Verification items for the finished model (mm, model axes). A direction names the side the tool comes from. Round coordinates to 2 decimals unless told otherwise and drop trailing zeros. Order: outer loops, then holes, each group sorted by start corner. A loop starts at its lowest first (then second) coordinate and runs counter-clockwise, first axis right, second up. Notation, with made-up numbers: (21, 66) -> (32, 66) arc R19 ccw to (32, 95) -> close; hole circle Ø7 at (-9.75, 74). An arc over 180 degrees is marked (long way). Put each result on its own line as item: value.
Autodesk Inventor part; units mm, degrees
ref_plane "Work Plane1" through (-20, 20, -22) normal (0, -0.791285, -0.6114475) x (1, 0, 0)
ref_plane "YZ Plane" through (0, 0, 0) normal (1, 0, 0) x (0, 1, 0)
ref_plane "XZ Plane" through (0, 0, 0) normal (0, 1, 0) x (-1, 0, 0)
sketch "Sketch1" plane through (0, 0, 0) normal (0, 1, 0) x (-1, 0, 0)
  line L0 (0, 0) -> (20, 0)
  line L1 (20, 0) -> (20, -25)
  line L2 (20, -25) -> (0, -25)
  line L3 (0, -25) -> (0, 0)
  circle A0 centre (10, -11) radius 2.6
  line L4 (20, -25) -> (0, -25)
  line L5 (0, -25) -> (0, -22)
  line L6 (0, -22) -> (20, -22)
  line L7 (20, -22) -> (20, -25)
  line L8 (0, -22) -> (20, 0) construction
  point P0 (10, -11)
  dimension "d2" = 20
  dimension "d3" = 25
  dimension "d4" = 5.2
  dimension "d7" = 3
extrude "Extrusion1" add sketch "Sketch1" along normal blind 3
extrude "Extrusion2" add sketch "Sketch1" along normal blind 20 contours L6 L1 L2 L3
sketch "Sketch2" plane through (0, 0, -25) normal (0, 0, -1) x (-1, 0, 0)
  line L0 (0, 0) -> (0, 20)
  line L1 (20, 0) -> (20, 20)
  line L2 (0, 20) -> (20, 0) construction
  circle A0 centre (10, 10) radius 2.65
  dimension "d10" = 5.3
extrude "Extrusion3" cut sketch "Sketch2" against normal through all
ref_plane "Work Plane1" through (-20, 20, -22) normal (0, -0.791285, -0.6114475) x (1, 0, 0)
sketch "Sketch3" plane through (-20, 20, -22) normal (0, -0.791285, -0.6114475) x (1, 0, 0)
  line L0 (0, 27.8029) -> (20, 27.8029)
  line L1 (0, 0) -> (20, 0)
  line L2 (0, 10.3946) -> (0, 0)
  line L3 (0, 0) -> (3, 0)
  line L4 (3, 0) -> (3, 27.8029)
  line L5 (3, 27.8029) -> (0, 27.8029)
  line L6 (0, 27.8029) -> (0, 0)
  line L7 (20, 27.8029) -> (17, 27.8029)
  line L8 (17, 27.8029) -> (17, 0)
  line L9 (17, 0) -> (20, 0)
  line L10 (20, 0) -> (20, 27.8029)
  point P0 (20, 29.6372)
  point P1 (20, 0)
  dimension "d13" = 3
  dimension "d14" = 3
extrude "Extrusion4" add sketch "Sketch3" along normal up to next contours L0 L4 L1 L2 L6 | L0 L10 L1 L8
chamfer "Chamfer1" distance 2.75 angle 45 5 edges at (-10, 3, -22) (-3, 11.5, -22) (-3, 3, -11) (-17, 3, -11) (-17, 11.5, -22)
sketch "Sketch4" plane through (0, 0, 0) normal (0, -1, 0) x (1, 0, 0)
  line L0 (0, -25) -> (-20, -25)
  line L1 (-20, 0) -> (0, 0)
  line L2 (-14.375, -25) -> (-5.625, -25)
  line L3 (-5.625, -25) -> (-5.625, 0)
  line L4 (-5.625, 0) -> (-14.375, 0)
  line L5 (-14.375, 0) -> (-14.375, -25)
  circle A0 centre (-10, -11) radius 2.6
  line L6 (-10, -25) -> (-10, 0) construction
  line L7 (-5.625, -6) -> (-14.375, -6)
  line L8 (-14.375, -6) -> (-14.375, -16)
  line L9 (-14.375, -16) -> (-5.625, -16)
  line L10 (-5.625, -16) -> (-5.625, -6)
  line L11 (-14.375, -16) -> (-5.625, -6) construction
  point P0 (-14.375, 0)
  dimension "d32" = 8.75
  dimension "d42" = 10
extrude "Extrusion5" add sketch "Sketch4" along normal blind 1.35 contours L0 L5 L9 L3 | L7 L5 L1 L3
sketch "Sketch5" plane through (0, 20, -25) normal (0, 0, -1) x (-1, 0, 0)
  line L0 (0, 0) -> (0, -17)
  line L1 (20, -17) -> (20, 0)
  line L2 (0, -5.625) -> (20, -5.625)
  line L3 (20, -5.625) -> (20, -14.375)
  line L4 (20, -14.375) -> (0, -14.375)
  line L5 (0, -14.375) -> (0, -5.625)
  line L6 (0, -14.375) -> (20, -5.625) construction
  circle A0 centre (10, -10) radius 2.65
  line L7 (5, -5.625) -> (15, -5.625)
  line L8 (15, -5.625) -> (15, -14.375)
  line L9 (15, -14.375) -> (5, -14.375)
  line L10 (5, -14.375) -> (5, -5.625)
  line L11 (5, -5.625) -> (15, -14.375) construction
  point P0 (0, -20)
  point P1 (0, -14.375)
  point P2 (5, -14.375)
  dimension "d26" = 8.75
  dimension "d43" = 10
extrude "Extrusion6" add sketch "Sketch5" along normal blind 1.35 contours L2 L10 L4 L0 | L2 L1 L4 L8
chamfer "Chamfer2" distance 1.35 angle 45 8 edges at (-17.5, 5.625, -26.35) (-2.5, 5.625, -26.35) (-17.5, 14.375, -26.35) (-2.5, 14.375, -26.35) (-14.375, -1.35, -3) (-14.375, -1.35, -20.5) (-5.625, -1.35, -3) (-5.625, -1.35, -20.5)
sketch "Sketch9" plane through (-20, 0, -25) normal (-1, 0, 0) x (0, 0, 1)
  line L0 (-1.35, 6.975) -> (-1.35, 13.025)
  line L1 (0, 0) -> (0, 5.625)
  line L2 (0, 0) -> (25, 0)
  line L3 (25, 0) -> (25, 3)
  line L4 (25, 3) -> (3, 20)
  line L5 (0, 20) -> (3, 20)
  line L6 (0, 14.375) -> (0, 20)
  line L7 (0, 14.375) -> (4.4808, 18.8558)
  line L8 (-1.35, 13.025) -> (0, 14.375)
  line L9 (0, 5.625) -> (-1.35, 6.975)
  point P0 (25, 0)
extrude "Extrusion10" add sketch "Sketch9" along normal blind 10 contours L6 L5 L4 L7
fillet "Fillet2" radius 3 1 edges at (-20, 16.6154, -22.7596)
properties part number "Soporte Actuador MIR" material "PET Plastic"
Item 1: Sectioned sample at A-A, the plane z = -11. Record the boundary of the cut face in (x, y), then the cut area to 3 significant figures.
Geometry check:
outline: (-20, 0) -> (-12.6, 0) -> (-12.6, 3) -> (-14.25, 3) -> (-17, 5.75) -> (-17, 11.5) -> (-20, 11.5) -> close; (-7.4, 0) -> (0, 0) -> (0, 11.5) -> (-3, 11.5) -> (-3, 5.75) -> (-5.75, 3) -> (-7.4, 3) -> close
area: 103 mm2
Item 2: Tool access check on faces 1 (the face through (-19.17, 12.72, -12.58)), 2 (the face through (-10, -1, -16)), 3 (the face through (-15.64, 4.39, -9.49)), 4 (the face through (-5, 10, -26)), 5 (the face through (-10, -1.35, -20)). Record the directions out of +Z, -Z, +X, -X, +Y, -Y that give a thin tool (end or side, any length) a straight path to the whole face; none if there is none.
Geometry check:
face 1: +Z, +X, -X, +Y
face 2: +X, -X, -Y
face 3: +Z, +Y
face 4: -Z, +Y, -Y
face 5: +Z, -Z, +X, -X, -Y
Item 3: Material ranges on line 1 along X through (y, z) = (12, -18.25); line 2 along Y through (x, z) = (-10, -23.35); line 3 along Z through (x, y) = (-16, 2.25), recorded low to high.
Geometry check:
line 1: -20 to -17, -3 to 0
line 2: -1.35 to 7.35, 12.65 to 20
line 3: -25 to 0
Item 4: Depth check by flat-ended pin: pin 1 Ø2.5 at (x, y) = (-12, 12.5) entering from +Z; pin 2 Ø7 at (x, y) = (-10, 10) entering from -Z; pin 3 Ø0.7 at (y, z) = (9, -25.5) entering from -X. Enter the tip coordinate at first touch or a pass-through.
Geometry check:
pin 1: z = -22
pin 2: z = -25
pin 3: x = -20
Item 5: Release check for a two-part mould opening along X. For faces 6 (the face through (-1.637, 11.381, -10.846)), 7 (the face through (-10, 3, -7)), 8 (the face through (-6.291, -0.666, -20.563)) record: pulls with the +X half, pulls with the -X half, needs draft (parallel to the pull), parting line crosses it, or undercut.
Geometry check:
face 6: needs draft
face 7: undercut
face 8: pulls with the +X half
Item 6: Sectioned sample at C-C, the plane x = -10. Record the boundary of the cut face in (y, z).
Geometry check:
outline: (-1.35, -25) -> (7.35, -25) -> (7.35, -22) -> (5.75, -22) -> (3, -19.25) -> (3, -13.6) -> (0, -13.6) -> (0, -16) -> (-1.35, -16) -> close; (-1.35, -6) -> (0, -6) -> (0, -8.4) -> (3, -8.4) -> (3, 0) -> (-1.35, 0) -> close; (12.65, -25) -> (20, -25) -> (20, -22) -> (12.65, -22) -> close
